from build123d import *

# Parameters (mm, degrees)
SKETCH1_W           = 105.3
SKETCH1_H           = 45.3
SKETCH1_R           = 18.65
BOSS_EXTRUDE1_DEPTH = 20
SKETCH2_W           = 105.3
SKETCH2_H           = 45.3
SKETCH2_R           = 6.15
SKETCH2_R_2         = 1.5
BOSS_EXTRUDE2_DEPTH = 4
SKETCH3_W           = 11
SKETCH3_H           = 24
SKETCH3_R           = 2
BOSS_EXTRUDE3_DEPTH = 5
FILLET1_R           = 2
BOSS_EXTRUDE4_START = -5
SKETCH4_W           = 11
SKETCH4_H           = 24
SKETCH4_R           = 2
BOSS_EXTRUDE4_DEPTH = 5
FILLET2_R           = 2
SKETCH6_R           = 4
CUT_EXTRUDE1_DEPTH  = 20
SKETCH7_R           = 4.047183171
CUT_EXTRUDE2_DEPTH  = 20
SKETCH8_R           = 4
CUT_EXTRUDE3_DEPTH  = 20


with BuildPart() as part:
    # Sketch1 → Boss-Extrude1 (new body)
    with BuildSketch(Plane.XY):
        with Locations((30, 0)):
            Rectangle(SKETCH1_W, SKETCH1_H)
        Circle(SKETCH1_R, mode=Mode.SUBTRACT)
        with Locations(Location((60, 0, 0), (0, 0, 180))):
            Circle(SKETCH1_R, mode=Mode.SUBTRACT)
    extrude(amount=-BOSS_EXTRUDE1_DEPTH)

    # Sketch2 → Boss-Extrude2 (add)
    with BuildSketch(Plane.XY):
        with Locations((30, 0)):
            Rectangle(SKETCH2_W, SKETCH2_H)
        with Locations((-8, 0)):
            Circle(SKETCH2_R, mode=Mode.SUBTRACT)
        with Locations((0, 15.25)):
            Circle(SKETCH2_R_2, mode=Mode.SUBTRACT)
        with Locations((13.206887408, 7.625)):
            Circle(SKETCH2_R_2, mode=Mode.SUBTRACT)
        with Locations((13.206887408, -7.625)):
            Circle(SKETCH2_R_2, mode=Mode.SUBTRACT)
        with Locations((0, -15.25)):
            Circle(SKETCH2_R_2, mode=Mode.SUBTRACT)
        with Locations((-13.206887408, -7.625)):
            Circle(SKETCH2_R_2, mode=Mode.SUBTRACT)
        with Locations((-13.206887408, 7.625)):
            Circle(SKETCH2_R_2, mode=Mode.SUBTRACT)
        with Locations(Location((73.206887408, -7.625, 0), (0, 0, 180))):
            Circle(SKETCH2_R_2, mode=Mode.SUBTRACT)
        with Locations(Location((60, -15.25, 0), (0, 0, 180))):
            Circle(SKETCH2_R_2, mode=Mode.SUBTRACT)
        with Locations(Location((46.793112592, -7.625, 0), (0, 0, 180))):
            Circle(SKETCH2_R_2, mode=Mode.SUBTRACT)
        with Locations(Location((46.793112592, 7.625, 0), (0, 0, 180))):
            Circle(SKETCH2_R_2, mode=Mode.SUBTRACT)
        with Locations(Location((60, 15.25, 0), (0, 0, 180))):
            Circle(SKETCH2_R_2, mode=Mode.SUBTRACT)
        with Locations(Location((73.206887408, 7.625, 0), (0, 0, 180))):
            Circle(SKETCH2_R_2, mode=Mode.SUBTRACT)
        with Locations(Location((68, 0, 0), (0, 0, 180))):
            Circle(SKETCH2_R, mode=Mode.SUBTRACT)
    extrude(amount=BOSS_EXTRUDE2_DEPTH)

    # Sketch3 → Boss-Extrude3 (add)
    # profile 1 of 2: a face of its own
    with BuildSketch(Plane.XZ.offset(22.65)):
        with Locations((-28.15, -8)):
            Rectangle(SKETCH3_W, SKETCH3_H)
        with Locations(Location((-29.65, -4, 0), (0, 0, 270))):
            Circle(SKETCH3_R, mode=Mode.SUBTRACT)
        with Locations(Location((-29.65, -12, 0), (0, 0, 270))):
            Circle(SKETCH3_R, mode=Mode.SUBTRACT)
    # profile 2 of 2: a face of its own
    with BuildSketch(Plane.XZ.offset(22.65)):
        with Locations((88.15, -8)):
            Rectangle(SKETCH3_W, SKETCH3_H)
        with Locations(Location((89.65, -4, 0), (0, 0, 90))):
            Circle(SKETCH3_R, mode=Mode.SUBTRACT)
        with Locations(Location((89.65, -12, 0), (0, 0, 90))):
            Circle(SKETCH3_R, mode=Mode.SUBTRACT)
    extrude(amount=-BOSS_EXTRUDE3_DEPTH)

    # Fillet1
    fillet1_edges = [part.edges().sort_by_distance(p)[0] for p in [
        (-22.65, -17.65, -8),
        (82.65, -17.65, -8),
    ]]
    fillet(fillet1_edges, radius=FILLET1_R)

    # Sketch4 → Boss-Extrude4 (add)
    # profile 1 of 2: a face of its own
    with BuildSketch(Plane(origin=(0, 22.65, 0), x_dir=(1, 0, 0), z_dir=(0, 1, 0)).offset(BOSS_EXTRUDE4_START)):
        with Locations((-28.15, 8)):
            Rectangle(SKETCH4_W, SKETCH4_H)
        with Locations(Location((-29.65, 12, 0), (0, 0, 90))):
            Circle(SKETCH4_R, mode=Mode.SUBTRACT)
        with Locations(Location((-29.65, 4, 0), (0, 0, 90))):
            Circle(SKETCH4_R, mode=Mode.SUBTRACT)
    # profile 2 of 2: a face of its own
    with BuildSketch(Plane(origin=(0, 22.65, 0), x_dir=(1, 0, 0), z_dir=(0, 1, 0)).offset(BOSS_EXTRUDE4_START)):
        with Locations((88.15, 8)):
            Rectangle(SKETCH4_W, SKETCH4_H)
        with Locations(Location((89.65, 12, 0), (0, 0, 270))):
            Circle(SKETCH4_R, mode=Mode.SUBTRACT)
        with Locations(Location((89.65, 4, 0), (0, 0, 270))):
            Circle(SKETCH4_R, mode=Mode.SUBTRACT)
    extrude(amount=BOSS_EXTRUDE4_DEPTH)

    # Fillet2
    fillet2_edges = [part.edges().sort_by_distance(p)[0] for p in [
        (-22.65, 17.65, -8),
        (82.65, 17.65, -8),
    ]]
    fillet(fillet2_edges, radius=FILLET2_R)

    # Sketch6 → Cut-Extrude1 (cut)
    with BuildSketch(Plane.XZ.offset(22.65)):
        with Locations((2.5, -22.368602792)):
            Circle(SKETCH6_R)
        with Locations((2.5, -117.631397208)):
            Circle(SKETCH6_R)
    extrude(amount=-CUT_EXTRUDE1_DEPTH, mode=Mode.SUBTRACT)

    # Sketch7 → Cut-Extrude2 (cut)
    with BuildSketch(Plane.XZ.offset(22.65)):
        with Locations((2.5, -22.368602792)):
            Circle(SKETCH7_R)
    extrude(amount=-CUT_EXTRUDE2_DEPTH, mode=Mode.SUBTRACT)

    # Sketch8 → Cut-Extrude3 (cut)
    with BuildSketch(Plane(origin=(0, 22.65, 0), x_dir=(1, 0, 0), z_dir=(0, 1, 0))):
        with Locations((2.5, 22.368602792)):
            Circle(SKETCH8_R)
    extrude(amount=-CUT_EXTRUDE3_DEPTH, mode=Mode.SUBTRACT)


solid = part.part
The listing builds one solid part. Answer for the finished solid, in the listing's coordinates (mm). A direction names the side the tool comes from. Coordinates: 2 decimals unless noted, no trailing zeros. Loops run counter-clockwise (first coordinate to the right, second up) from the corner with the lowest first, then second, coordinate; pieces in that order, holes last. Notation, with made-up numbers: M 86,40 L 109,40 A21 cw 109,70 Z; hole C 58.5,89.5 d9. An arc over 180 degrees is marked long. Answer in a Markdown table with one row per item.
1) Given pin 1 (1.8 mm diameter, centred on x = 73.21, y = -7.62, fed in from +Z); pin 2 (5 mm diameter, centred on y = 1, z = 0.5, fed in from +X); pin 3 (11 mm diameter, centred on x = 8.5, y = -0.5, fed in from -Z); pin 4 (2 mm diameter, centred on y = -12, z = -1, fed in from -X), each flat-ended and moving along its own axis, determine where each tip first touches the part or whether it passes through.
Answers below:
| item | result |
|---|---|
| pin 1 | through |
| pin 2 | x = 82.65 |
| pin 3 | z = 0 |
| pin 4 | x = -22.65 |
2) Determine the mould class of faces 5 (the flat face through (0, 0, 0)), 6 (the cylindrical face through (87.698, 20.115, -4.434)) for opening direction Y: released by +Y, released by -Y, zero draft, split by the parting line, or undercut.
Answers below:
| item | result |
|---|---|
| face 5 | undercut |
| face 6 | zero draft |
3) Find section C-C (y = 0). Determine the outline of the cut face in (x, z).
Answers below:
| item | result |
|---|---|
| outline | M -22.65,-20 L -18.65,-20 L -18.65,0 L -14.15,0 L -14.15,4 L -22.65,4 Z; M -1.85,0 L 18.65,0 L 18.65,-20 L 41.35,-20 L 41.35,0 L 61.85,0 L 61.85,4 L -1.85,4 Z; M 74.15,0 L 78.65,0 L 78.65,-20 L 82.65,-20 L 82.65,4 L 74.15,4 Z |
4) Find section B-B (x = 89.65). Determine the outline of the cut face in (y, z), then the cut area to 3 significant figures.
Answers below:
| item | result |
|---|---|
| outline | M -22.65,-20 L -17.65,-20 L -17.65,-14 L -22.65,-14 Z; M -22.65,-10 L -17.65,-10 L -17.65,-6 L -22.65,-6 Z; M -22.65,-2 L -17.65,-2 L -17.65,4 L -22.65,4 Z; M 17.65,-20 L 22.65,-20 L 22.65,-14 L 17.65,-14 Z; M 17.65,-10 L 22.65,-10 L 22.65,-6 L 17.65,-6 Z; M 17.65,-2 L 22.65,-2 L 22.65,4 L 17.65,4 Z |
| area | 160 mm^2 |
5) Find section A-A (z = -3.75). Count the separate pieces of the cut face and the enclosed holes in it, then the cut area to 3 significant figures.
Answers below:
| item | result |
|---|---|
| separate pieces | 5 |
| enclosed holes | 2 |
| area | 2,730 mm^2 |
6) Find section D-D (x = -9.5). Determine the outline of the cut face in (y, z).
Answers below:
| item | result |
|---|---|
| outline | M -22.65,-20 L -16.05,-20 L -16.05,0 L -5.96,0 L -5.96,4 L -22.65,4 Z; M 5.96,0 L 16.05,0 L 16.05,-20 L 22.65,-20 L 22.65,4 L 5.96,4 Z |
7) Find the intervals of material crossed by probe 1 along X at (y, z) = (19.9, -12); probe 2 along X at (y, z) = (-13, -15.25); probe 3 along Y at (x, z) = (-25, 2.5), in increasing order.
Answers below:
| item | result |
|---|---|
| probe 1 | -33.65 to -31.65, -27.65 to 87.65, 91.65 to 93.65 |
| probe 2 | -22.65 to -13.37, 13.37 to 46.63, 73.37 to 82.65 |
| probe 3 | -22.65 to -17.65, 17.65 to 22.65 |
8) Which of the six approach directions +Z, -Z, +X, -X, +Y, -Y give full straight-line access (tool end or side, diameter ignored) to faces 1 (the flat face through (-22.65, 0, -8)), 2 (the flat face through (82.65, 0, -8)), 3 (the cylindrical face through (78.63, -0.82, -9.86)), 4 (the cylindrical face through (91.602, -20.185, -12.434))?
Answers below:
| item | result |
|---|---|
| face 1 | +Z, -Z, -X |
| face 2 | +Z, -Z, +X |
| face 3 | -Z |
| face 4 | +Y, -Y |
